from build123d import *

# Parameters (mm, degrees)
F0_W     = 152.4
F0_H     = 101.6
F1_DEPTH = 127
F2_R     = 12.7
F3_W     = 53.302623
F3_H     = 31.648196
F4_DEPTH = 12.7


with BuildPart() as f1:
    # F0 (on Top) → F1 (new body)
    with BuildSketch(Plane.XY):
        with Locations((14.119559, -8.696024)):
            Rectangle(F0_W, F0_H)
    extrude(amount=F1_DEPTH)

    # F2
    f2_edges = [f1.edges().sort_by_distance(p)[0] for p in [
        (14.119559, -59.496024, 127),
    ]]
    fillet(f2_edges, radius=F2_R)

    # F3 (on face) → F4 (cut)
    with BuildSketch(Plane.XZ.offset(59.496024)):
        with Locations((10.842934, 70.015054)):
            Rectangle(F3_W, F3_H)
    extrude(amount=-F4_DEPTH, mode=Mode.SUBTRACT)


solid = f1.part
Build history of the part. All positions in model axes, mm. A direction names the side the tool comes from. Round coordinates to 2 decimals unless told otherwise and drop trailing zeros. Write each loop counter-clockwise with the first axis right and the second up, starting at its lowest first coordinate (ties: lowest second). Pieces come first, ordered by that corner, then holes. Notation, with made-up numbers: M -24,38 L -12,38 A30 ccw -12,65 Z; hole C 24,75 d2. An arc over 180 degrees is marked long. Answer in a Markdown table with one row per item.
1. Mould opens along Z. For faces 3 (the face through (15.186, -55.874, 123.181)), 4 (the face through (90.32, -9, 63)), 5 (the face through (10, -46.796, 70)), 6 (the face through (13, -8, 0)) say: +Z half, -Z half, draft (parallel to the pull), parting line (faces both ways), or undercut.
Geometry check:
| item | result |
|---|---|
| face 3 | +Z half |
| face 4 | draft |
| face 5 | undercut |
| face 6 | -Z half |
2. Saw through at A-A (x = 20.5). List the corners of the cut face in (y, z), and give its area (3 significant figures).
Geometry check:
| item | result |
|---|---|
| outline | M -59.5,0 L 42.1,0 L 42.1,127 L -46.8,127 A12.7 ccw -59.5,114.3 L -59.5,85.84 L -46.8,85.84 L -46.8,54.19 L -59.5,54.19 Z |
| area | 12,500 mm2 |
3. Probe L1, parallel to Y at x = 17, z = 65; L2, parallel to Z at x = -24, y = -52; L3, parallel to Z at x = 60, y = -48. List the from-to ranges inside material, lowest first. Write a range as [from, to].
Geometry check:
| item | result |
|---|---|
| L1 | [-46.8, 42.1] |
| L2 | [0, 125.88] |
| L3 | [0, 126.94] |
4. Which spindle directions (+Z, -Z, +X, -X, +Y, -Y) get a long thin tool onto all of the face, cutting with end or side? Do faces 1 (the face through (13, -2, 127)), 2 (the face through (10, -53, 54.191)). Say none if no direction does.
Geometry check:
| item | result |
|---|---|
| face 1 | +Z, +X, -X, +Y, -Y |
| face 2 | -Y |
5. Saw through at B-B (z = 81). List the corners of the cut face in (x, y), and give its area (3 significant figures).
Geometry check:
| item | result |
|---|---|
| outline | M -62.08,-59.5 L -15.81,-59.5 L -15.81,-46.8 L 37.49,-46.8 L 37.49,-59.5 L 90.32,-59.5 L 90.32,42.1 L -62.08,42.1 Z |
| area | 14,800 mm2 |
